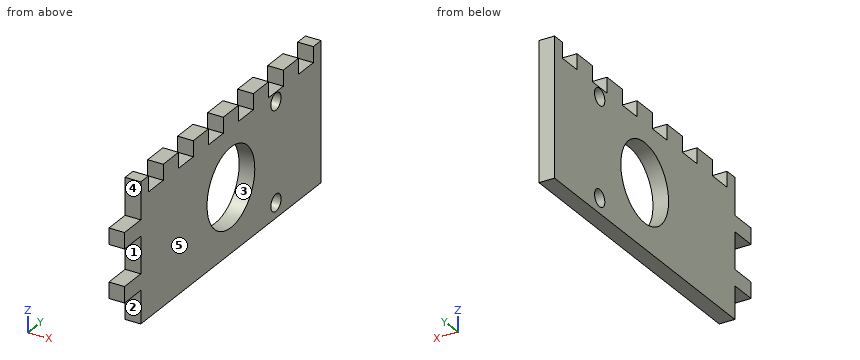
```python
from build123d import *

# Parameters (mm, degrees)
SKETCH1_W           = 24.825
SKETCH1_H           = 3.175
SKETCH1_W_2         = 3.175
SKETCH1_H_2         = 24.825
BOSS_EXTRUDE1_DEPTH = 60
SKETCH2_W           = 3.125
SKETCH2_H           = 5.4
BOSS_EXTRUDE4_DEPTH = 3.175
SKETCH4_R           = 8
CUT_EXTRUDE1_DEPTH  = 3.175
SKETCH3_R           = 8
CUT_EXTRUDE2_DEPTH  = 3.175
SKETCH5_W           = 3.175
SKETCH5_H           = 5.4
BOSS_EXTRUDE5_DEPTH = 3.175
SKETCH6_R           = 1.75
CUT_EXTRUDE3_DEPTH  = 10
SKETCH7_R           = 1.75
CUT_EXTRUDE4_DEPTH  = 10
SKETCH9_W           = 3.175
SKETCH9_H           = 65.4
CUT_EXTRUDE5_DEPTH  = 24.825
SKETCH10_W          = 3.175
SKETCH10_H          = 5
CUT_EXTRUDE6_DEPTH  = 10
SKETCH11_R          = 7.95936
SKETCH11_R_2        = 1.70936
BOSS_EXTRUDE6_DEPTH = 3.175


with BuildPart() as part:
    # Sketch1 → Boss-Extrude1 (new body)
    with BuildSketch(Plane(origin=(0, 0, 0), x_dir=(1, 0, 0), z_dir=(0, 1, 0))):
        with Locations((-38.0875, 24.0875)):
            Rectangle(SKETCH1_W, SKETCH1_H)
        with Locations((-24.0875, 24.0875)):
            Rectangle(SKETCH1_W_2, SKETCH1_H)
        with Locations((-24.0875, 38.0875)):
            Rectangle(SKETCH1_W_2, SKETCH1_H_2)
    extrude(amount=BOSS_EXTRUDE1_DEPTH)

    # Sketch2 → Boss-Extrude4 (add)
    with BuildSketch(Plane.XY.offset(-22.5)):
        with Locations((-42.1875, -2.7)):
            Rectangle(SKETCH2_W, SKETCH2_H)
        with Locations((-31.5625, -2.7)):
            Rectangle(SKETCH2_W, SKETCH2_H)
    extrude(amount=-BOSS_EXTRUDE4_DEPTH)

    # Sketch4 → Cut-Extrude1 (cut)
    with BuildSketch(Plane.XY.offset(-22.5)):
        with Locations((-37.5, 30)):
            Circle(SKETCH4_R)
    extrude(amount=-CUT_EXTRUDE1_DEPTH, mode=Mode.SUBTRACT)

    # Sketch3 → Cut-Extrude2 (cut)
    with BuildSketch(Plane(origin=(-22.5, 0, 0), x_dir=(0, 0, -1), z_dir=(1, 0, 0))):
        with Locations((37.5, 30)):
            Circle(SKETCH3_R)
    extrude(amount=-CUT_EXTRUDE2_DEPTH, mode=Mode.SUBTRACT)

    # Sketch5 → Boss-Extrude5 (add)
    with BuildSketch(Plane(origin=(-22.5, 0, 0), x_dir=(0, 0, -1), z_dir=(1, 0, 0))):
        with Locations((42.2625, -2.7)):
            Rectangle(SKETCH5_W, SKETCH5_H)
        with Locations((31.5875, -2.7)):
            Rectangle(SKETCH5_W, SKETCH5_H)
    extrude(amount=-BOSS_EXTRUDE5_DEPTH)

    # Sketch6 → Cut-Extrude3 (cut)
    with BuildSketch(Plane.XY.offset(-22.5)):
        with Locations((-47.5, 45)):
            Circle(SKETCH6_R)
        with Locations((-27.5, 45)):
            Circle(SKETCH6_R)
    extrude(amount=-CUT_EXTRUDE3_DEPTH, mode=Mode.SUBTRACT)

    # Sketch7 → Cut-Extrude4 (cut)
    with BuildSketch(Plane(origin=(-22.5, 0, 0), x_dir=(0, 0, -1), z_dir=(1, 0, 0))):
        with Locations((47.5, 45)):
            Circle(SKETCH7_R)
        with Locations((27.5, 45)):
            Circle(SKETCH7_R)
    extrude(amount=-CUT_EXTRUDE4_DEPTH, mode=Mode.SUBTRACT)

    # Sketch9 → Cut-Extrude5 (cut)
    with BuildSketch(Plane.ZY.offset(50.5)):
        with Locations((-24.0875, 27.3)):
            Rectangle(SKETCH9_W, SKETCH9_H)
    extrude(amount=-CUT_EXTRUDE5_DEPTH, mode=Mode.SUBTRACT)

    # Sketch10 → Cut-Extrude6 (cut)
    with BuildSketch(Plane.ZY.offset(25.675)):
        with Locations((-24.0875, 55)):
            Rectangle(SKETCH10_W, SKETCH10_H)
        with Locations((-24.0875, 45)):
            Rectangle(SKETCH10_W, SKETCH10_H)
        with Locations((-24.0875, 35)):
            Rectangle(SKETCH10_W, SKETCH10_H)
        with Locations((-24.0875, 25)):
            Rectangle(SKETCH10_W, SKETCH10_H)
        with Locations((-24.0875, 15)):
            Rectangle(SKETCH10_W, SKETCH10_H)
        with Locations((-24.0875, 5)):
            Rectangle(SKETCH10_W, SKETCH10_H)
    extrude(amount=-CUT_EXTRUDE6_DEPTH, mode=Mode.SUBTRACT)

    # Sketch11 → Boss-Extrude6 (add)
    with BuildSketch(Plane(origin=(-22.5, 0, 0), x_dir=(0, 0, -1), z_dir=(1, 0, 0))):
        Polygon((25.63436, 57.45936), (25.63436, 52.54064), (22.45936, 52.54064), (22.45936, 47.45936), (25.63436, 47.45936), (25.63436, 42.54064), (22.45936, 42.54064), (22.45936, 37.45936), (25.63436, 37.45936), (25.63436, 32.54064), (22.45936, 32.54064), (22.45936, 27.45936), (25.63436, 27.45936), (25.63436, 22.54064), (22.45936, 22.54064), (22.45936, 17.45936), (25.63436, 17.45936), (25.63436, 12.54064), (22.45936, 12.54064), (22.45936, 7.45936), (25.63436, 7.45936), (25.63436, 2.54064), (22.45936, 2.54064), (22.45936, -0.04064), (29.95936, -0.04064), (29.95936, -5.44064), (33.21564, -5.44064), (33.21564, -0.04064), (40.63436, -0.04064), (40.63436, -5.44064), (43.89064, -5.44064), (43.89064, -0.04064), (50.54064, -0.04064), (50.54064, 60.04064), (22.45936, 60.04064), (22.45936, 57.45936), align=None)
        with Locations((37.5, 30)):
            Circle(SKETCH11_R, mode=Mode.SUBTRACT)
        with Locations((27.5, 45)):
            Circle(SKETCH11_R_2, mode=Mode.SUBTRACT)
        with Locations((47.5, 45)):
            Circle(SKETCH11_R_2, mode=Mode.SUBTRACT)
    extrude(amount=-BOSS_EXTRUDE6_DEPTH)


solid = part.part
```
Geometry check sheet. Reference: the model listing, model coordinates, mm. Face numbers are marked on the shaded views. A direction names the side the tool comes from. Round coordinates to 2 decimals unless told otherwise and drop trailing zeros. Order: outer loops, then holes, each group sorted by start corner. A loop starts at its lowest first (then second) coordinate and runs counter-clockwise, first axis right, second up. Notation, with made-up numbers: M 26,-10 L 34,-10 A29 cw 34,11 Z; hole C 16.25,55 d9. An arc over 180 degrees is marked long. Write item = value, one per line.
Q1. Section check A-A (y = 45). Enter the section's corners in (x, z) (3 decimals).
Answer block:
outline = M -25.675,-50.541 L -22.5,-50.541 L -22.5,-49.209 L -25.675,-49.209 Z; M -25.675,-45.791 L -22.5,-45.791 L -22.5,-29.209 L -25.675,-29.209 Z; M -25.675,-25.791 L -22.5,-25.791 L -22.5,-25.634 L -25.675,-25.634 Z
Q2. Set-up check for the marked faces 4 and 5: record each of +Z, -Z, +X, -X, +Y, -Y from which the full face is reachable in a straight line by a thin tool's end or side.
Answer block:
face_4 = +Z, +X, -X, -Y
face_5 = +Z, -Z, +X, +Y, -Y
Q3. Scan lines: line 1 (Y direction, x = -23.65, z = -37.5); line 2 (Y direction, x = -23.3, z = -47.5); line 3 (Z direction, x = -23, y = 4). Record each from-to range of solid material in increasing order.
Answer block:
line_1 = -0.04 to 22.04, 37.96 to 60.04
line_2 = -0.04 to 43.29, 46.71 to 60.04
line_3 = -50.54 to -25.63
Q4. Section check D-D (x = -23.85). Give the number of separate pieces and of enclosed holes in the cut face, plus the area to 3 significant figures.
Answer block:
separate_pieces = 1
enclosed_holes = 3
area = 1,410 mm^2
Q5. Release check for a two-part mould opening along Z. For the marked faces 1, 2 and 3 record: released by +Z, released by -Z, zero draft, split by the parting line, or undercut.
Answer block:
face_1 = undercut
face_2 = zero draft
face_3 = undercut
Q6. Section check B-B (z = -27.5). Enter the section's corners in (x, y) (3 decimals), plus the area to 3 significant figures.
Answer block:
outline = M -25.675,-0.041 L -22.5,-0.041 L -22.5,43.291 L -25.675,43.291 Z; M -25.675,46.709 L -22.5,46.709 L -22.5,60.041 L -25.675,60.041 Z
area = 180 mm^2
Q7. Section check C-C (y = 30). Enter the section's corners in (x, z) (3 decimals), plus the area to 3 significant figures.
Answer block:
outline = M -25.675,-50.541 L -22.5,-50.541 L -22.5,-45.459 L -25.675,-45.459 Z; M -25.675,-29.541 L -22.5,-29.541 L -22.5,-22.459 L -25.675,-22.459 Z
area = 38.6 mm^2
Q8. Depth check by flat-ended pin: pin 1 Ø1 at (x, z) = (-23, -28.5) entering from -Y. Enter the tip coordinate at first touch or a pass-through.
Answer block:
pin_1 = -0.04
